from build123d import *

# Parameters (mm, degrees)
BOX_W           = 49.18
BOX_H           = 23.8
BOX_DEPTH       = 5
SKETCH_W        = 43.2
SKETCH_H        = 17.8
POCKET_DEPTH    = 2
SKETCH001_W     = 3
SKETCH001_H     = 9
POCKET001_DEPTH = 2
SKETCH004_R     = 1
POCKET005_DEPTH = 5
SKETCH005_R     = 1.51127
POCKET006_DEPTH = 5


with BuildPart() as part:
    # Box → Box (new body)
    with BuildSketch(Plane.XY):
        with Locations((24.59, 11.9)):
            Rectangle(BOX_W, BOX_H)
    extrude(amount=BOX_DEPTH)

    # Sketch → Pocket (cut)
    with BuildSketch(Plane.XY.offset(5)):
        with Locations((24.6, 11.9)):
            Rectangle(SKETCH_W, SKETCH_H)
    extrude(amount=-POCKET_DEPTH, mode=Mode.SUBTRACT)

    # Sketch001 → Pocket001 (cut)
    with BuildSketch(Plane.XY.offset(5)):
        with Locations((1.5, 11.9)):
            Rectangle(SKETCH001_W, SKETCH001_H)
    extrude(amount=-POCKET001_DEPTH, mode=Mode.SUBTRACT)

    # Sketch004 → Pocket005 (cut)
    with BuildSketch(Plane.XY.offset(3)):
        with Locations((44.722157, 19.634458)):
            Circle(SKETCH004_R)
        with Locations((44.722157, 4.622099)):
            Circle(SKETCH004_R)
        with Locations((4.133191, 19.634458)):
            Circle(SKETCH004_R)
        with Locations((4.133191, 4.622099)):
            Circle(SKETCH004_R)
    extrude(amount=-POCKET005_DEPTH, mode=Mode.SUBTRACT)

    # Sketch005 → Pocket006 (cut)
    with BuildSketch(Plane(origin=(0, 0, 0), x_dir=(1, 0, 0), z_dir=(0, 0, -1))):
        with Locations((10.59, -11.9)):
            Circle(SKETCH005_R)
        with Locations((38.59, -11.9)):
            Circle(SKETCH005_R)
    extrude(amount=-POCKET006_DEPTH, mode=Mode.SUBTRACT)


solid = part.part
Geometry: final body of the model. Coordinates: model frame, mm. A direction names the side the tool comes from. Give positions to 0.01 mm unless a question says otherwise; leave off trailing zeros. Write each loop counter-clockwise with the first axis right and the second up, starting at its lowest first coordinate (ties: lowest second). Pieces come first, ordered by that corner, then holes. Notation, with made-up numbers: (7, 21) -> (57, 21) arc R33 cw to (57, 57) -> close; hole circle Ø9 at (-6, 85). An arc over 180 degrees is marked (long way). Answer as a JSON object with one key per item and string values.
1. Cut plane A-A on y = 11.9. Output: boundary loops of the cut face in (x, z), and give its area (3 significant figures).
Ans:
{"outline": "(0, 0) -> (9.08, 0) -> (9.08, 3) -> (0, 3) -> close; (12.1, 0) -> (37.08, 0) -> (37.08, 3) -> (12.1, 3) -> close; (40.1, 0) -> (49.18, 0) -> (49.18, 5) -> (46.2, 5) -> (46.2, 3) -> (40.1, 3) -> close", "area": "135 mm^2"}
2. Cut plane B-B on x = 38.59. Output: boundary loops of the cut face in (y, z).
Ans:
{"outline": "(0, 0) -> (10.39, 0) -> (10.39, 3) -> (3, 3) -> (3, 5) -> (0, 5) -> close; (13.41, 0) -> (23.8, 0) -> (23.8, 5) -> (20.8, 5) -> (20.8, 3) -> (13.41, 3) -> close"}
3. Ray query, probe 1 along X at (y, z) = (11.9, 1.45); probe 2 along Y at (x, z) = (26, 3.65); probe 3 along Y at (x, z) = (38.59, 1.65). Return the intervals inside material, ascending. Write a range as from..to.
Ans:
{"probe 1": "x = 0..9.08, 12.1..37.08, 40.1..49.18", "probe 2": "y = 0..3, 20.8..23.8", "probe 3": "y = 0..10.39, 13.41..23.8"}
4. Cut plane D-D on z = 3.8. Output: boundary loops of the cut face in (x, y), and give its area (3 significant figures).
Ans:
{"outline": "(0, 0) -> (49.18, 0) -> (49.18, 23.8) -> (0, 23.8) -> (0, 16.4) -> (3, 16.4) -> (3, 20.8) -> (46.2, 20.8) -> (46.2, 3) -> (3, 3) -> (3, 7.4) -> (0, 7.4) -> close", "area": "375 mm^2"}
5. Contact query for flat-ended pins moving along their axis: pin 1 (1.2 mm diameter, centred on x = 44.72, y = 19.63, fed in from +Z); pin 2 (3 mm diameter, centred on x = 8.5, y = 14.5, fed in from -Z). Output: stop coordinate, or through.
Ans:
{"pin 1": "passes through", "pin 2": "stops at z = 0"}
6. Access query for faces 4 (the flat face through (1, 7.4, 4)), 5 (the cylindrical face through (11.402, 10.626, 1.479)), 6 (the flat face through (24, 3, 4)). Directions: +Z, -Z, +X, -X, +Y, -Y. A direction counts if a zero-diameter tool reaches every point of the face in a straight line with its end or side. Return the directions, or none.
Ans:
{"face 4": "+Z, -X", "face 5": "+Z, -Z", "face 6": "+Z"}
7. Cut plane C-C on x = 28. Output: boundary loops of the cut face in (y, z).
Ans:
{"outline": "(0, 0) -> (23.8, 0) -> (23.8, 5) -> (20.8, 5) -> (20.8, 3) -> (3, 3) -> (3, 5) -> (0, 5) -> close"}
8. Mould query, pull axis Y, two halves, no side actions, for faces 1 (the flat face through (24, 23.8, 2)), 2 (the flat face through (24, 12, 0)), 3 (the flat face through (3, 19, 4)). Classes: pulls with the +Y half, pulls with the -Y half, needs draft (parallel to the pull), parting line crosses it, or undercut.
Ans:
{"face 1": "pulls with the +Y half", "face 2": "needs draft", "face 3": "undercut"}
